```python
from build123d import *

# Parameters (mm, degrees)
SKETCH1_R               = 100
BOSS_EXTRUDE1_DEPTH     = 75
BOSS_EXTRUDE1_TAPER     = 7.5
CUT_EXTRUDE1_DEPTH      = 125
CUT_EXTRUDE1_DEPTH_BACK = 122
SKETCH3_R               = 7.673209678
BOSS_EXTRUDE5_DEPTH     = 15
SKETCH5_R               = 25
CUT_EXTRUDE3_DEPTH      = 12.5
SKETCH6_R               = 62.5
CUT_EXTRUDE4_DEPTH      = 22.5


with BuildPart() as part:
    # Sketch1 → Boss-Extrude1 (new body)
    with BuildSketch(Plane(origin=(0, 0, 0), x_dir=(1, 0, 0), z_dir=(0, 1, 0))):
        Circle(SKETCH1_R)
    extrude(amount=BOSS_EXTRUDE1_DEPTH, taper=BOSS_EXTRUDE1_TAPER)

    # Sketch2 → Cut-Extrude1 (cut, two sides: drawn at the far end of the back side and taken through both)
    with BuildSketch(Plane(origin=(0, 0, 0), x_dir=(0, 0, -1), z_dir=(1, 0, 0)).offset(-CUT_EXTRUDE1_DEPTH_BACK)):
        with BuildLine():
            Line((-12.527814818, 45), (12.472185182, 45))
            ThreePointArc((12.472185182, 45), (19.972185182, 37.5), (12.472185182, 30))
            Line((12.472185182, 30), (-12.527814818, 30))
            ThreePointArc((-12.527814818, 30), (-20.027814818, 37.5), (-12.527814818, 45))
        make_face()
    extrude(amount=CUT_EXTRUDE1_DEPTH + CUT_EXTRUDE1_DEPTH_BACK, mode=Mode.SUBTRACT)

    # Sketch3 → Boss-Extrude5 (add, symmetric)
    with BuildSketch(Plane.XY):
        with Locations((94.960632329, 37.526119935)):
            Circle(SKETCH3_R)
    boss_extrude5 = extrude(amount=BOSS_EXTRUDE5_DEPTH, both=True)

    # Mirror1: Boss-Extrude5 across plane
    add(boss_extrude5.mirror(Plane(origin=(0, 0, 0), x_dir=(0, 0, 1), z_dir=(1, 0, 0))))

    # Sketch5 → Cut-Extrude3 (cut)
    with BuildSketch(Plane.XZ):
        with Locations(Location((0, 0, 0), (0, 0, 270))):
            Circle(SKETCH5_R)
    extrude(amount=-CUT_EXTRUDE3_DEPTH, mode=Mode.SUBTRACT)

    # Sketch6 → Cut-Extrude4 (cut)
    with BuildSketch(Plane(origin=(0, 12.5, 0), x_dir=(1, 0, 0), z_dir=(0, 1, 0))):
        with Locations(Location((0, 0, 0), (0, 0, 18.22154092))):
            Circle(SKETCH6_R)
    extrude(amount=CUT_EXTRUDE4_DEPTH, mode=Mode.SUBTRACT)


solid = part.part
```
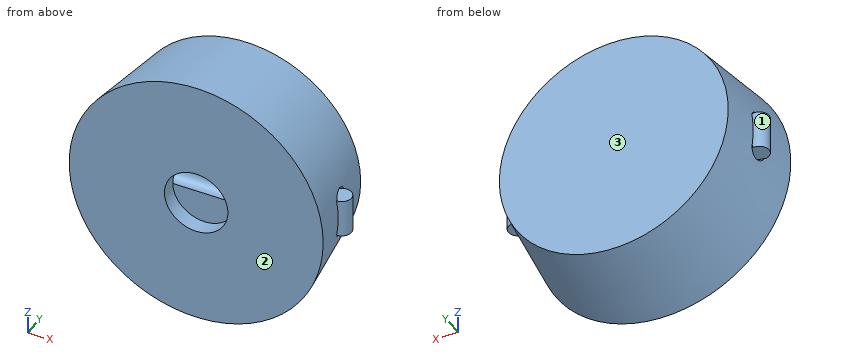
The model under review builds one solid part; all positions refer to its coordinate system, in mm. Face numbers are marked on the shaded views. Coordinates: 2 decimals unless noted, no trailing zeros. Write each loop counter-clockwise with the first axis right and the second up, starting at its lowest first coordinate (ties: lowest second). Pieces come first, ordered by that corner, then holes. Notation, with made-up numbers: (87, -19.75) -> (141, -19.75) arc R19 ccw to (141, 2.25) -> close; hole circle Ø6 at (33.25, -29.5). An arc over 180 degrees is marked (long way). One line per item, written item: value. Start each with the question number.
Q1. The part is to be moulded in two halves that separate along Y. For the marked faces 1, 2 and 3, say which applies: +Y half, -Y half, draft (parallel to the pull), parting line (faces both ways), or undercut.
Q2. Add section C-C, the plane y = 69. Give the boundary of the cut face in (x, z).
Q3. To check wall thickness, follow probe 1 along Y at (x, z) = (-18, 28); probe 2 along Y at (x, z) = (53.5, 11); probe 3 along Z at (x, y) = (17, 12). State the ranges of each line that lie inside material, in increasing order.
Q4. Add section A-A, the plane x = 0. Give the boundary of the cut face in (y, z).
Q5. Add section B-B, the plane y = 37.5. Give the boundary of the cut face in (x, z).
Q6. Clearance check with flat-ended pins moving along their axes: P1, Ø1.5, axis at y = 54.5, z = 17.5, coming from the -X side; P2, Ø6, axis at y = 66, z = 35, coming from the +X side; P3, Ø12, axis at y = 43, z = 63.5, coming from the +X side. State where each tip first meets the part, or that it passes through.
Response:
1. face 1: undercut
1. face 2: -Y half
1. face 3: +Y half
2. outline: circle Ø181.83 at (0, 0)
3. probe 1: 0 to 12.5, 35 to 75
3. probe 2: 0 to 12.5, 45 to 75
3. probe 3: -96.94 to -18.33, 18.33 to 96.94
4. outline: (0, -100) -> (75, -90.13) -> (75, 90.13) -> (0, 100) -> (0, 25) -> (12.5, 25) -> (12.5, 62.5) -> (35, 62.5) -> (35, 19.6) arc R7.5 cw to (45, 12.53) -> (45, -12.47) arc R7.5 cw to (35, -19.54) -> (35, -62.5) -> (12.5, -62.5) -> (12.5, -25) -> (0, -25) -> close
5. outline: (-102.63, -15) -> (-87.29, -15) -> (-87.29, 15) -> (-102.63, 15) -> close; (-92.94, -19.97) arc R95.06 ccw to (92.94, -19.97) -> close; (-92.93, 20.03) -> (92.93, 20.03) arc R95.06 ccw to start; (87.29, -15) -> (102.63, -15) -> (102.63, 15) -> (87.29, 15) -> close
6. P1: x = -91.33
6. P2: x = 85.6
6. P3: x = 74.9
